Answer from the drawing. Dimensions are ordinates in mm from the lowest x, y and z of the part. A direction names the side the tool comes from. Give positions to 0.01 mm unless a question says otherwise; leave off trailing zeros. Order: outer loops, then holes, each group sorted by start corner. A loop starts at its lowest first (then second) coordinate and runs counter-clockwise, first axis right, second up.
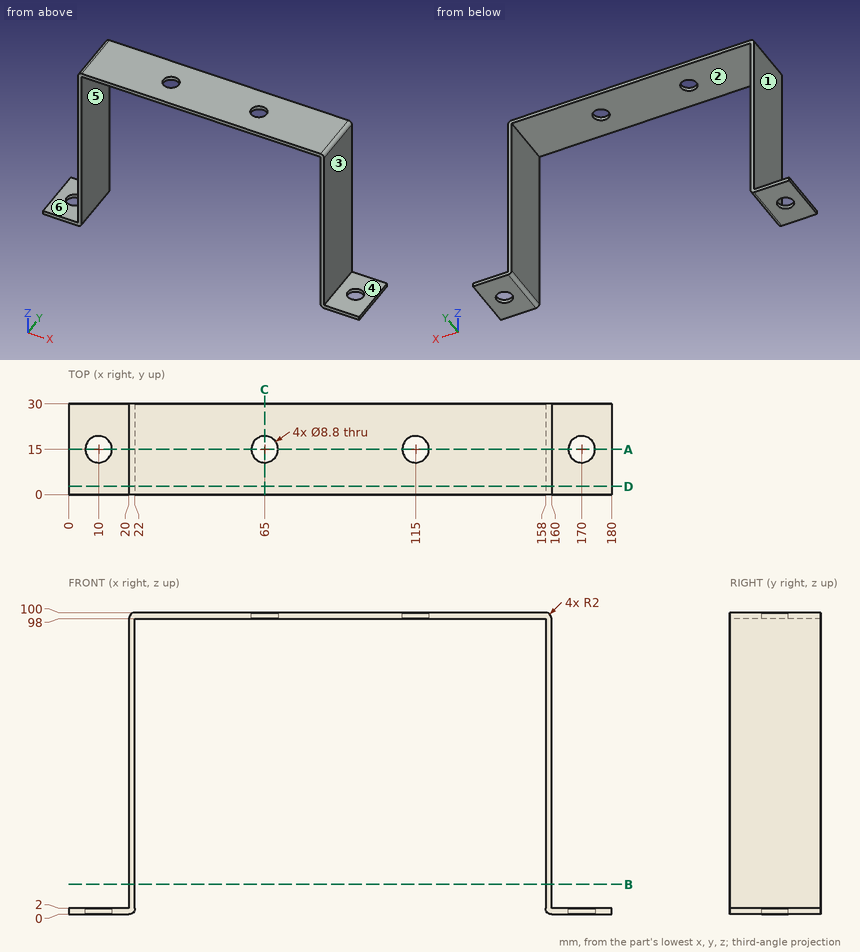
1) The part is cut by section C-C on x = 65. Determine the outline of the cut face in (y, z).
Final values:
outline: (0, 98) - (10.6, 98) - (10.6, 100) - (0, 100) - close; (19.4, 98) - (30, 98) - (30, 100) - (19.4, 100) - close
2) Consider L1, parallel to Y at x = 65, z = 99; L2, parallel to X at y = 8.25, z = 81; L3, parallel to Z at x = 51, y = 6. Determine where each line is inside the solid, lowest interval first.
Final values:
L1: y = 0 to 10.6, 19.4 to 30
L2: x = 20 to 22, 158 to 160
L3: z = 98 to 100
3) Given pin 1 (1.5 mm diameter, centred on x = 89, y = 24.5, fed in from -Z); pin 2 (15 mm diameter, centred on y = 8, z = 32, fed in from -X); pin 3 (8 mm diameter, centred on x = 65, y = 15, fed in from +Z); pin 4 (10 mm diameter, centred on x = 115, y = 15, fed in from +Z), each flat-ended and moving along its own axis, determine where each tip first touches the part or whether it passes through.
Final values:
pin 1: stops at z = 98
pin 2: stops at x = 20
pin 3: passes through
pin 4: stops at z = 100
4) For a pull along X with two mould halves and no side action, classify the marked faces 1, 2 and 3 as released by +X, released by -X, zero draft, split by the parting line, or undercut.
Final values:
face 1: released by -X
face 2: undercut
face 3: released by +X
5) The part is cut by section A-A on y = 15. Count the separate pieces of the cut face and the enclosed holes in it, and give its area (3 significant figures).
Final values:
separate pieces: 5
enclosed holes: 0
area: 678 mm2
6) The part is cut by section B-B on z = 10. Determine the outline of the cut face in (x, y), and give its area (3 significant figures).
Final values:
outline: (20, 0) - (22, 0) - (22, 30) - (20, 30) - close; (158, 0) - (160, 0) - (160, 30) - (158, 30) - close
area: 120 mm2
7) A tool of negligible diameter and unlimited length cuts with its end or side. For the marked faces 4, 5 and 6, from which of +Z, -Z, +X, -X, +Y, -Y can it reach the whole face along a straight path? Write none if from no direction.
Final values:
face 4: +Z, +X, +Y, -Y
face 5: -Z, +Y, -Y
face 6: +Z, -X, +Y, -Y
8) The part is cut by section D-D on y = 2.75. Determine the outline of the cut face in (x, z), and give its area (3 significant figures).
Final values:
outline: (0, 0) - (20, 0) arc R2 ccw to (22, 2) - (22, 98) - (158, 98) - (158, 2) arc R2 ccw to (160, 0) - (180, 0) - (180, 2) - (160, 2) - (160, 98) arc R2 ccw to (158, 100) - (22, 100) arc R2 ccw to (20, 98) - (20, 2) - (0, 2) - close
area: 749 mm2
